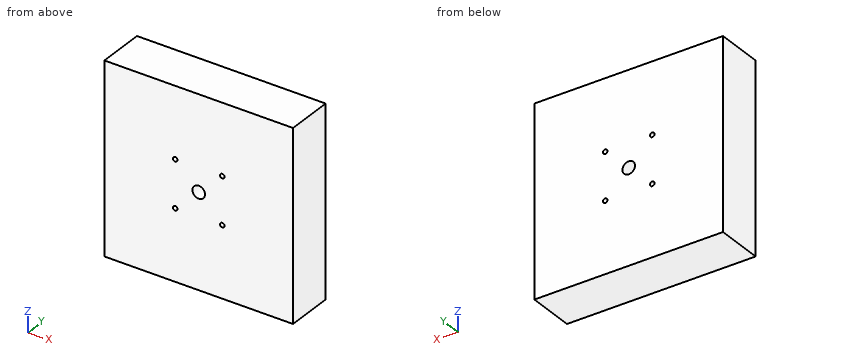
```python
from build123d import *

# Parameters (mm, degrees)
SKETCH1_W               = 101.6
SKETCH1_H               = 101.6
BOSS_EXTRUDE1_DEPTH     = 25.4
F_1_4_CLEARANCE_HOLE1_D = 6.7564
F_2_CLEARANCE_HOLE1_D   = 2.4384
F_2_CLEARANCE_HOLE2_D   = 2.4384


with BuildPart() as part:
    # Sketch1 → Boss-Extrude1 (new body)
    with BuildSketch(Plane(origin=(0, 0, 0), x_dir=(1, 0, 0), z_dir=(0, 1, 0))):
        Rectangle(SKETCH1_W, SKETCH1_H)
    extrude(amount=BOSS_EXTRUDE1_DEPTH)

    # 1/4 Clearance Hole1 (through all)
    with Locations(Plane(origin=(0, 25.4, 0), x_dir=(1, 0, 0), z_dir=(0, 1, 0))):
        with Locations((0, 0)):
            Hole(F_1_4_CLEARANCE_HOLE1_D / 2)

    # #2 Clearance Hole1 (through all)
    with Locations(Plane(origin=(0, 25.4, 0), x_dir=(1, 0, 0), z_dir=(0, 1, 0))):
        with Locations((-12.7, 12.7), (0, 0)):
            Hole(F_2_CLEARANCE_HOLE1_D / 2)

    # #2 Clearance Hole2 (through all)
    with Locations(Plane(origin=(0, 25.4, 0), x_dir=(1, 0, 0), z_dir=(0, 1, 0))):
        with Locations((12.7, 12.7), (-12.7, -12.7), (12.7, -12.7)):
            Hole(F_2_CLEARANCE_HOLE2_D / 2)


solid = part.part
```
Check sheet for the modelled part. Datum: model origin and axes. Units: mm. Coordinates: 2 decimals unless noted, no trailing zeros. Order: outer loops, then holes, each group sorted by start corner. A loop starts at its lowest first (then second) coordinate and runs counter-clockwise, first axis right, second up. Notation, with made-up numbers: (74.5, 73.5) -> (83.5, 73.5) arc R19 ccw to (83.5, 83.5) -> close; hole circle Ø2 at (18, 49). An arc over 180 degrees is marked (long way). Write item = value, one per line. Start each with the question number.
1) Cross-section at C-C (z = 12.7). Enter the section's corners in (x, y), then the cut area to 3 significant figures.
2) Material ranges on L1, parallel to Z at x = -12.7, y = 19.75; L2, parallel to Z at x = 0, y = 8.5, recorded low to high.
3) Cross-section at A-A (z = 0). Enter the section's corners in (x, y).
4) Cross-section at B-B (x = 12.7). Enter the section's corners in (y, z), then the cut area to 3 significant figures.
5) Go/stop test with a flat-tipped pin: P1, Ø1.5, axis at x = -12.7, z = -12.7, coming from the +Y side. Record where the tip stops, or that it passes through.
Ans:
q1.outline = (-50.8, 0) -> (-13.92, 0) -> (-13.92, 25.4) -> (-50.8, 25.4) -> close; (-11.48, 0) -> (11.48, 0) -> (11.48, 25.4) -> (-11.48, 25.4) -> close; (13.92, 0) -> (50.8, 0) -> (50.8, 25.4) -> (13.92, 25.4) -> close
q1.area = 2,460 mm²
q2.L1 = -50.8 to -13.92, -11.48 to 11.48, 13.92 to 50.8
q2.L2 = -50.8 to -3.38, 3.38 to 50.8
q3.outline = (-50.8, 0) -> (-3.38, 0) -> (-3.38, 25.4) -> (-50.8, 25.4) -> close; (3.38, 0) -> (50.8, 0) -> (50.8, 25.4) -> (3.38, 25.4) -> close
q4.outline = (0, -50.8) -> (25.4, -50.8) -> (25.4, -13.92) -> (0, -13.92) -> close; (0, -11.48) -> (25.4, -11.48) -> (25.4, 11.48) -> (0, 11.48) -> close; (0, 13.92) -> (25.4, 13.92) -> (25.4, 50.8) -> (0, 50.8) -> close
q4.area = 2,460 mm²
q5.P1 = through
